For this review, use the dimensioned drawing (mm, ordinates from the lowest corner) and the shaded views. Round coordinates to 2 decimals unless told otherwise and drop trailing zeros. Loops run counter-clockwise (first coordinate to the right, second up) from the corner with the lowest first, then second, coordinate; pieces in that order, holes last.
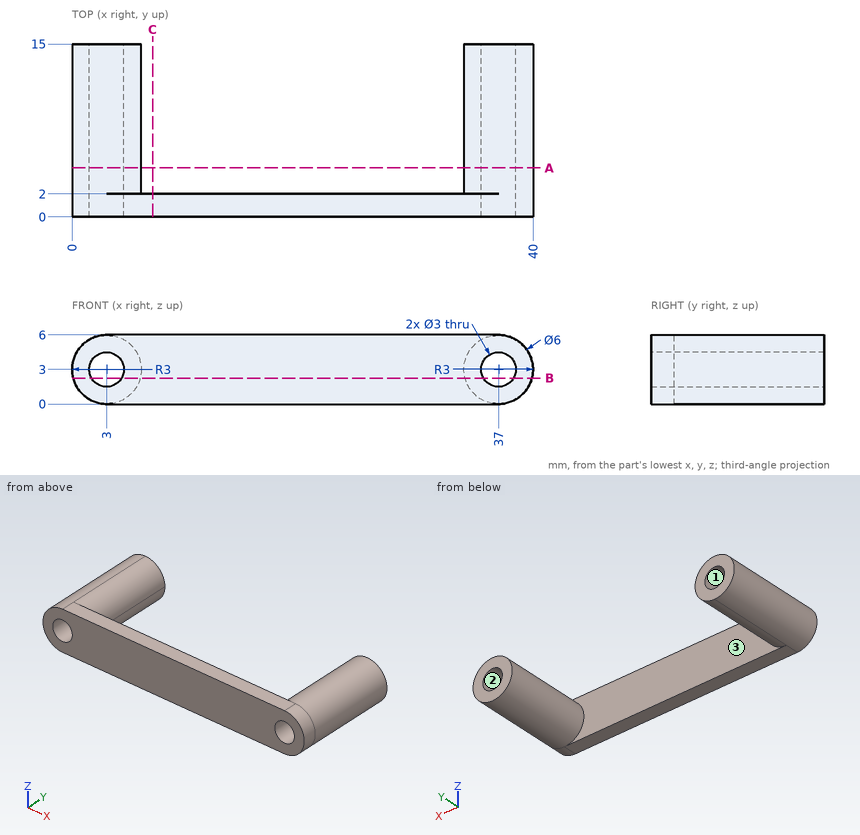
(1) Insertion check: pin 1 Ø8 at (x, y) = (32, 8) entering from +Z; pin 2 Ø3 at (x, y) = (34, 5.5) entering from -Z; pin 3 Ø1.5 at (y, z) = (11, 1) entering from +X. Each pin has a flat end and moves straight along its axis. Give the tip position at first contact, or say it passes through.
(2) Add section B-B (z = 2.25). Give the boundary of the cut face in (x, y), plus the area to 3 significant figures.
(3) Add section C-C (x = 7). Give the boundary of the cut face in (y, z), plus the area to 3 significant figures.
(4) For L1, parallel to Y at x = 25.5, z = 4; L2, parallel to X at y = 11.75, z = 2; L3, parallel to X at y = 9.25, z = 4.75, list the stretches that pass through material, from the lowest coordinate up.
(5) The part is to be moulded in two halves that separate along Z. For the marked faces 1, 2 and 3, say which applies: pulls with the +Z half, pulls with the -Z half, needs draft (parallel to the pull), parting line crosses it, or undercut.
(6) Add section A-A (y = 4.25). Give the boundary of the cut face in (x, z), plus the area to 3 significant figures.
Outcome:
1. pin 1: stops at z = 5.83
1. pin 2: stops at z = 0.4
1. pin 3: stops at x = 39.73
2. outline: (0.1, 0) - (1.7, 0) - (1.7, 15) - (0.1, 15) - close; (4.3, 0) - (35.7, 0) - (35.7, 15) - (34.1, 15) - (34.1, 2) - (5.9, 2) - (5.9, 15) - (4.3, 15) - close; (38.3, 0) - (39.9, 0) - (39.9, 15) - (38.3, 15) - close
2. area: 153 mm2
3. outline: (0, 0) - (2, 0) - (2, 6) - (0, 6) - close
3. area: 12.0 mm2
4. L1: y = 0 to 2
4. L2: x = 0.17 to 1.88, 4.12 to 5.83, 34.17 to 35.88, 38.12 to 39.83
4. L3: x = 0.56 to 5.44, 34.56 to 39.44
5. face 1: undercut
5. face 2: undercut
5. face 3: needs draft
6. outline: circle Ø6 at (3, 3); circle Ø6 at (37, 3); hole circle Ø3 at (3, 3); hole circle Ø3 at (37, 3)
6. area: 42.4 mm2
